For this review, take the finished solid that the model builds, in its own axes (mm). A direction names the side the tool comes from. Coordinates: 2 decimals unless noted, no trailing zeros. Loops run counter-clockwise (first coordinate to the right, second up) from the corner with the lowest first, then second, coordinate; pieces in that order, holes last. Notation, with made-up numbers: (70.5, 88) - (124.5, 88) arc R29 cw to (124.5, 115) - close; hole circle Ø10 at (60, 62.25). An arc over 180 degrees is marked (long way). One line per item, written item: value. Start each with the question number.
1. Take a section at C-C, the plane x = 1.5. State the section outline as (y, z) points.
2. For faces 1 (the face through (0, 0, 0)), 2 (the face through (11.944, 3.905, 0.867)), 3 (the face through (6, 0, 3)), list the 3-axis set-ups (+Z, -Z, +X, -X, +Y, -Y) from which the entire face can be reached by the end or side of a thin tool; tool diameter is ignored.
3. Take a section at A-A, the plane y = 0. State the section outline as (x, z) points, and give its area (3 significant figures).
4. Take a section at D-D, the plane x = 6.5. State the section outline as (y, z) points.
5. To check wall thickness, follow line 1 (X direction, y = -9.25, z = 8.25); line 2 (X direction, y = 3.25, z = 1.5); line 3 (Z direction, x = 4.25, y = 3.25). State the ranges of each line that lie inside material, in increasing order. Write a range as from..to.
6. Insertion check: pin 1 (3 mm diameter, centred on x = 13.5, z = 6.5, fed in from -Y); pin 2 (1.5 mm diameter, centred on x = 5, y = 8, fed in from +Z); pin 3 (5 mm diameter, centred on x = 14.5, y = 4, fed in from +Z); pin 4 (4 mm diameter, centred on y = 1.5, z = 10, fed in from -X). Each pin has a flat end and moves straight along its axis. Give the tip position at first contact, or say it passes through.
Autodesk Inventor part; units mm, degrees
ref_plane "YZ Plane" through (0, 0, 0) normal (1, 0, 0) x (0, 1, 0)
ref_plane "XZ Plane" through (0, 0, 0) normal (0, 1, 0) x (-1, 0, 0)
ref_plane "XY Plane" through (0, 0, 0) normal (0, 0, 1) x (1, 0, 0)
sketch "草圖1" plane through (0, 0, 0) normal (1, 0, 0) x (0, 1, 0)
  circle A0 centre (0, 0) radius 14
  dimension "d0" = 28
extrude "擠出1" add sketch "草圖1" along normal blind 5
sketch "草圖2" plane through (5, 0, 0) normal (1, 0, 0) x (0, 0, -1)
  circle A0 centre (0, 0) radius 3
  dimension "d3" = 6
extrude "擠出2" add sketch "草圖2" along normal blind 3
sketch "草圖3" plane through (8, 0, 0) normal (1, 0, 0) x (0, 0, -1)
  circle A0 centre (0, 0) radius 4
  dimension "d6" = 8
extrude "擠出3" add sketch "草圖3" along normal blind 9
chamfer "倒角1" distance 1 angle 45 3 edges at (17, 0, 4) (5, -14, 0) (0, -14, 0)
thread "螺紋1"
properties part number "2. 螺栓"
Solutions:
1. outline: circle Ø28 at (0, 0)
2. face 1: +Z, -Z, -X, +Y, -Y
2. face 2: +X
2. face 3: none
3. outline: (0, -13) - (1, -14) - (4, -14) - (5, -13) - (5, -3) - (8, -3) - (8, -4) - (16, -4) - (17, -3) - (17, 3) - (16, 4) - (8, 4) - (8, 3) - (5, 3) - (5, 13) - (4, 14) - (1, 14) - (0, 13) - close
3. area: 227 mm2
4. outline: circle Ø6 at (0, 0)
5. line 1: 0..5
5. line 2: 0..5, 8..16.42
5. line 3: -13.36..13.36
6. pin 1: through
6. pin 2: z = 11.32
6. pin 3: z = 3.71
6. pin 4: x = 0
